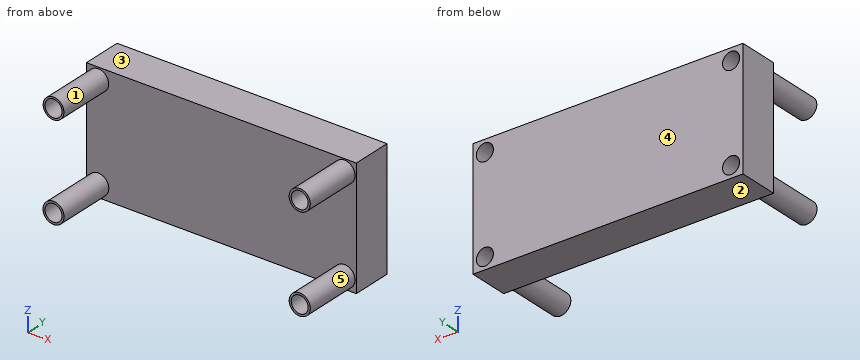
from build123d import *

# Parameters (mm, degrees)
SKETCH1_W           = 51.943
SKETCH1_H           = 22.8092
BOSS_EXTRUDE1_DEPTH = 7.6962
SKETCH2_R           = 1.9939
SKETCH2_R_2         = 2.032
BOSS_EXTRUDE2_DEPTH = 11.2268
SKETCH3_R           = 1.6383
CUT_EXTRUDE1_DEPTH  = 19.923


with BuildPart() as part:
    # Sketch1 → Boss-Extrude1 (new body)
    with BuildSketch(Plane(origin=(0, 0, 0), x_dir=(1, 0, 0), z_dir=(0, 1, 0))):
        with Locations((9.107555138, 0.071457393)):
            Rectangle(SKETCH1_W, SKETCH1_H)
    extrude(amount=BOSS_EXTRUDE1_DEPTH)

    # Sketch2 → Boss-Extrude2 (add)
    with BuildSketch(Plane.XZ):
        with Locations((-14.577944862, 9.047142607)):
            Circle(SKETCH2_R)
        with Locations((32.793055138, 9.047142607)):
            Circle(SKETCH2_R_2)
        with Locations((32.793055138, -9.190057393)):
            Circle(SKETCH2_R_2)
        with Locations((-14.577944862, -9.190057393)):
            Circle(SKETCH2_R_2)
    extrude(amount=BOSS_EXTRUDE2_DEPTH)

    # Sketch3 → Cut-Extrude1 (cut, through all)
    with BuildSketch(Plane.XZ.offset(11.2268)):
        with Locations((-14.577944862, 9.047142607)):
            Circle(SKETCH3_R)
        with Locations((-14.577944862, -9.190057393)):
            Circle(SKETCH3_R)
        with Locations((32.793055138, -9.190057393)):
            Circle(SKETCH3_R)
        with Locations((32.793055138, 9.047142607)):
            Circle(SKETCH3_R)
    extrude(amount=-CUT_EXTRUDE1_DEPTH, mode=Mode.SUBTRACT)


solid = part.part
For this review, take the finished solid that the model builds, in its own axes (mm). Face numbers are marked on the shaded views. A direction names the side the tool comes from. Give positions to 0.01 mm unless a question says otherwise; leave off trailing zeros. Loops run counter-clockwise (first coordinate to the right, second up) from the corner with the lowest first, then second, coordinate; pieces in that order, holes last. Notation, with made-up numbers: M 22,6 L 31,6 A30 cw 31,42 Z; hole C 73.25,87 d8. An arc over 180 degrees is marked long. Answer as a JSON object with one key per item and string values. Group by question number.
Q1. Insertion check: P1, Ø5, axis at x = 21.5, y = -3, coming from the -Z side; P2, Ø11.5, axis at x = 9, z = 2, coming from the -Y side. Each pin has a flat end and moves straight along its axis. Give the tip position at first contact, or say it passes through.
Q2. Add section A-A on z = 8. Give the boundary of the cut face in (x, y), and give its area (3 significant figures).
Q3. Add section C-C on y = 6.25. Give the boundary of the cut face in (x, z).
Q4. Tool access review of the marked faces 1 and 2: name each direction out of +Z, -Z, +X, -X, +Y, -Y from which nothing blocks a thin tool from reaching the whole face with its end or side.
Q5. For probe 1 along X at (y, z) = (3.25, -9); probe 2 along X at (y, z) = (2, -7.75); probe 3 along Y at (x, z) = (17.5, -4.5), list the stretches that pass through material, from the lowest coordinate up. Write a range as [from, to].
Q6. Mouldability with a two-part tool opening along Z and no side actions: class the marked faces 3, 4 and 5 as +Z half, -Z half, draft (parallel to the pull), parting line (faces both ways), or undercut.
Q7. Add section B-B on y = -1.5. Give the boundary of the cut face in (x, z), and give its area (3 significant figures).
Q8. Add section D-D on x = 10.5. Give the boundary of the cut face in (y, z), and give its area (3 significant figures).
Checked values:
{
 "1": {"P1": "through", "P2": "y = 0"},
 "2": {"outline": "M -16.86,0 L -16.27,0 L -16.27,-11.23 L -15.84,-11.23 L -15.84,7.7 L -16.86,7.7 Z; M -13.32,-11.23 L -12.88,-11.23 L -12.88,0 L 31.05,0 L 31.05,-11.23 L 31.53,-11.23 L 31.53,7.7 L -13.32,7.7 Z; M 34.05,-11.23 L 34.53,-11.23 L 34.53,0 L 35.08,0 L 35.08,7.7 L 34.05,7.7 Z", "area": "382 mm²"},
 "3": {"outline": "M -16.86,-11.48 L 35.08,-11.48 L 35.08,11.33 L -16.86,11.33 Z; hole C -14.58,-9.19 d3.28; hole C -14.58,9.05 d3.28; hole C 32.79,-9.19 d3.28; hole C 32.79,9.05 d3.28"},
 "4": {"face 1": "-Y", "face 2": "-Z, +X, -X, +Y, -Y"},
 "5": {"probe 1": "[-16.86, -16.21], [-12.95, 31.17], [34.42, 35.08]", "probe 2": "[-16.86, -15.36], [-13.8, 32.01], [33.57, 35.08]", "probe 3": "[0, 7.7]"},
 "6": {"face 3": "+Z half", "face 4": "draft", "face 5": "undercut"},
 "7": {"outline": "C -14.58,-9.19 d4.06; C -14.58,9.05 d3.99; C 32.79,-9.19 d4.06; C 32.79,9.05 d4.06; hole C -14.58,-9.19 d3.28; hole C -14.58,9.05 d3.28; hole C 32.79,-9.19 d3.28; hole C 32.79,9.05 d3.28", "area": "17.7 mm²"},
 "8": {"outline": "M 0,-11.48 L 7.7,-11.48 L 7.7,11.33 L 0,11.33 Z", "area": "176 mm²"}
}
